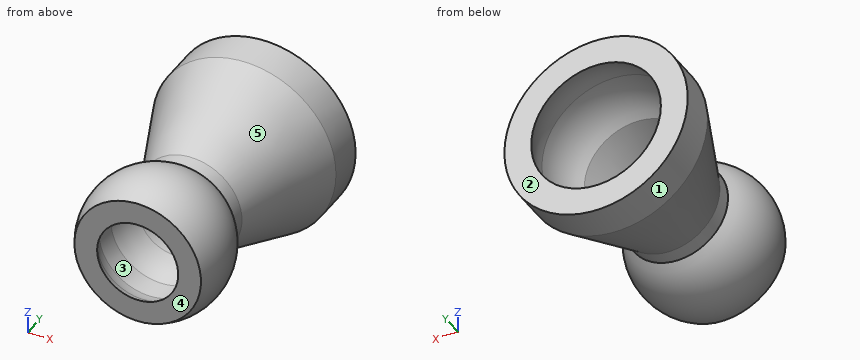
```python
from build123d import *


with BuildPart() as part:
    # Croquis1 → Revolución1 (revolve)
    with BuildSketch(Plane.XY):
        with BuildLine():
            Line((2.288621504, 0), (0, 0))
            Line((0, 0), (0, -3.17))
            Line((0, -3.17), (3.465, -11.76))
            Line((3.465, -11.76), (5.165, -11.76))
            Line((5.165, -11.76), (5.165, -11.43004663))
            Line((5.165, -11.43004663), (3.2627067, -6.714116055))
            ThreePointArc((3.2627067, -6.714116055), (2.140427602, -4.914602613), (1.7, -2.84004663))
            ThreePointArc((1.7, -2.84004663), (1.823561842, -1.38463429), (2.288621504, 0))
        make_face()
        with BuildLine():
            Line((5.165, -11.76), (3.465, -11.76))
            Line((3.465, -11.76), (3.465, -13.06))
            Line((3.465, -13.06), (4.667081528, -14.262081528))
            ThreePointArc((4.667081528, -14.262081528), (4.908103346, -14.038251376), (5.165, -13.83283579))
            Line((5.165, -13.83283579), (5.165, -11.76))
        make_face()
        with BuildLine():
            Line((4.667081528, -14.262081528), (3.465, -13.06))
            Line((3.465, -13.06), (3.465, -16.464646325))
            ThreePointArc((3.465, -16.464646325), (3.907580372, -15.276881881), (4.667081528, -14.262081528))
        make_face()
        with BuildLine():
            Line((3.465, -16.464646325), (3.465, -13.06))
            ThreePointArc((3.465, -13.06), (1.725988008, -16.53567688), (2.418118888, -20.36))
            Line((2.418118888, -20.36), (3.465, -20.36))
            Line((3.465, -20.36), (3.465, -18.352767084))
            ThreePointArc((3.465, -18.352767084), (3.363706704, -17.408706704), (3.465, -16.464646325))
        make_face()
        with BuildLine():
            Line((3.465, -18.352767084), (3.465, -16.464646325))
            ThreePointArc((3.465, -16.464646325), (3.363706704, -17.408706704), (3.465, -18.352767084))
        make_face()
        with BuildLine():
            ThreePointArc((3.909582187, -19.544195349), (3.644512403, -18.964444111), (3.465, -18.352767084))
            Line((3.465, -18.352767084), (3.465, -20.36))
            Line((3.465, -20.36), (4.355813233, -20.36))
            Line((4.355813233, -20.36), (3.909582187, -19.544195349))
        make_face()
    revolve(axis=Axis((7.813706704, 0, 0), (0, -1, 0)))


solid = part.part
```
Here's how the part is built. I have some questions about the finished solid (model axes, mm). Face numbers are marked on the shaded views. A direction names the side the tool comes from. Round coordinates to 2 decimals unless told otherwise and drop trailing zeros. Write each loop counter-clockwise with the first axis right and the second up, starting at its lowest first coordinate (ties: lowest second). Pieces come first, ordered by that corner, then holes. Notation, with made-up numbers: M 31,-31 L 90,-31 A16 ccw 90,-12 Z; hole C -21,50.5 d9. An arc over 180 degrees is marked long. Answer as CSV lines item,"result". Start each with the question number.
1. Suppose I cut it at A-A on y = -12.5. Write out the boundary of the cut face in (x, z) (3 decimals), then the cut area to 3 significant figures.
2. Suppose I cut it at B-B on z = 5.75. Count the separate pieces of the cut face and the enclosed holes in it, then the cut area to 3 significant figures.
3. I need wall thicknesses on probe 1 along X at (y, z) = (-12.05, 0) (3 decimals); probe 2 along Z at (x, y) = (8, -4); probe 3 along Z at (x, y) = (9.5, -4.25). Which ranges of each line are inside material? Lowest first, please.
4. I'm going to push flat-ended pins straight in: pin 1 Ø3 at (y, z) = (-11.5, 3) entering from -X; pin 2 Ø3 at (y, z) = (-15, 5.5) entering from +X; pin 3 Ø1.5 at (y, z) = (-16, 1) entering from -X; pin 4 Ø5 at (x, z) = (7.81, 0) entering from -Y. Where does each tip first touch, or does it pass through?
5. Suppose I cut it at C-C on y = -3.5. Write out the boundary of the cut face in (x, z).
6. On a 3-axis mill with a long thin cutter (end or side, diameter ignored), from which of +Z, -Z, +X, -X, +Y, -Y can I reach the whole of each face in a straight line? I mean the marked faces 4 and 5. Say none if no direction works.
7. Thinking about a two-plate mould opening in Z: for the marked faces 1, 2 and 3, which applies, released by +Z, released by -Z, zero draft, split by the parting line, or undercut?
Check result:
1,outline,"C 7.814,0 d8.697; hole C 7.814,0 d5.297"
1,area,"37.4 mm2"
2,separate pieces,"2"
2,enclosed holes,"1"
2,area,"69.8 mm2"
3,probe 1,"x = 3.465 to 5.165, 10.462 to 12.162"
3,probe 2,"z = -7.48 to -5.96, 5.96 to 7.48"
3,probe 3,"z = -7.18 to -5.65, 5.65 to 7.18"
4,pin 1,"stops at x = 3.33"
4,pin 2,"stops at x = 12"
4,pin 3,"stops at x = 1.74"
4,pin 4,"passes through"
5,outline,"C 7.81,0 d15.36; hole C 7.81,0 d12.11"
6,face 4,"+Z, -Z, +X, -X, -Y"
6,face 5,"none"
7,face 1,"split by the parting line"
7,face 2,"zero draft"
7,face 3,"undercut"
